Autodesk Inventor part; units mm, degrees
ref_plane "YZ Plane" through (0, 0, 0) normal (1, 0, 0) x (0, 1, 0)
ref_plane "XZ Plane" through (0, 0, 0) normal (0, 1, 0) x (-1, 0, 0)
ref_plane "XY Plane" through (0, 0, 0) normal (0, 0, 1) x (1, 0, 0)
sketch "Sketch1" plane through (0, 0, 0) normal (1, 0, 0) x (0, 1, 0)
  circle A0 centre (0, 0) radius 2.45
  dimension "d0" = 4.9
extrude "Extrusion1" add sketch "Sketch1" along normal blind 15
sketch "Sketch2" plane through (15, 0, 0) normal (1, 0, 0) x (0, 0, -1)
  circle A0 centre (0, 0) radius 2.45
  line L0 (-1.228, 2.12) -> (1.228, 2.12)
  dimension "d6" = 0.33
extrude "Extrusion2" cut sketch "Sketch2" against normal blind 8 contours L0 A0 picked at (-0.0856, 2.2255)
chamfer "Chamfer1" distance 0.5 angle 45 3 edges at (15, -2.45, 0) (0, -2.45, 0) (15, 2.12, 0)
properties part number "parrallelShaftPin"
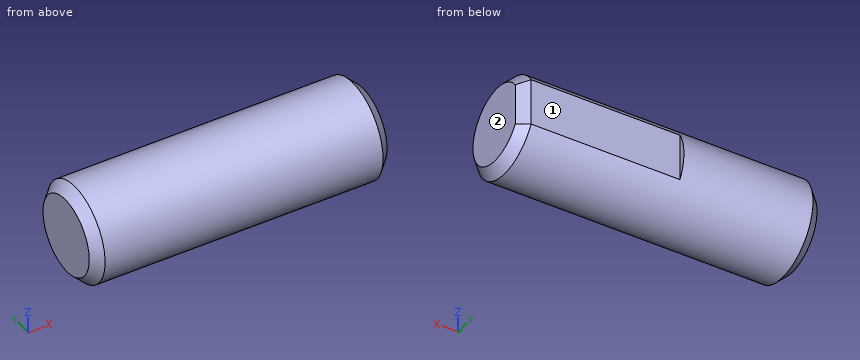
Source: CAD feature listing. Evaluate the final solid. Frame: model axes, mm. Face numbers are marked on the shaded views. A direction names the side the tool comes from. Round coordinates to 2 decimals unless told otherwise and drop trailing zeros. Loops run counter-clockwise (first coordinate to the right, second up) from the corner with the lowest first, then second, coordinate; pieces in that order, holes last. Notation, with made-up numbers: M 65.25,-1.5 L 90.25,-1.5 A20 ccw 90.25,24.5 Z; hole C 86,63.25 d7. An arc over 180 degrees is marked long. Use a Markdown table: item, result. Add a question column.
1. Section query B-B on x = 4. Return the cut outline in (y, z), then the cut area to 3 significant figures.
2. Contact query for flat-ended pins moving along their axis: P1, Ø2, axis at x = 13, z = -1.5, coming from the +Y side; P2, Ø1, axis at x = 7, z = 1.5, coming from the -Y side. Output: stop coordinate, or through.
3. Reachability of the marked faces 1 and 2 from +Z, -Z, +X, -X, +Y, -Y: full face, straight path, thin tool, end or side. Return the list, or none.
4. Section query C-C on x = 10.75. Return the cut outline in (y, z), then the cut area to 3 significant figures.
5. Section query A-A on z = 0. Return the cut outline in (x, y), then the cut area to 3 significant figures.
6. Line query: line 1 (Z direction, x = 13, y = -1.2); line 2 (X direction, y = 1.8, z = 1); line 3 (Z direction, x = 7.75, y = -1.45). Output: solid intervals per line, ascending.
Reported:
| question | item | result |
|---|---|---|
| 1 | outline | C 0,0 d4.9 |
| 1 | area | 18.9 mm² |
| 2 | P1 | stops at y = 2.12 |
| 2 | P2 | stops at y = -2.24 |
| 3 | face 1 | +Z, -Z, +X, +Y |
| 3 | face 2 | +Z, -Z, +X, +Y, -Y |
| 4 | outline | M 2.12,-1.23 L 2.12,1.23 A2.45 ccw long Z |
| 4 | area | 18.3 mm² |
| 5 | outline | M 0,-1.95 L 0.5,-2.45 L 14.5,-2.45 L 15,-1.95 L 15,1.62 L 14.5,2.12 L 7,2.12 L 7,2.45 L 0.5,2.45 L 0,1.95 Z |
| 5 | area | 70.4 mm² |
| 6 | line 1 | z = -2.14 to 2.14 |
| 6 | line 2 | x = 0.11 to 14.82 |
| 6 | line 3 | z = -1.97 to 1.97 |
